Model file for the job. Use its own axes, mm. Face numbers are marked on the shaded views. A direction names the side the tool comes from. Round coordinates to 2 decimals unless told otherwise and drop trailing zeros. Loops run counter-clockwise (first coordinate to the right, second up) from the corner with the lowest first, then second, coordinate; pieces in that order, holes last. Notation, with made-up numbers: (77.25, -7) -> (89.25, -7) arc R11 cw to (89.25, 3) -> close; hole circle Ø5 at (76, 31.5). An arc over 180 degrees is marked (long way). Use a Markdown table: item, result.
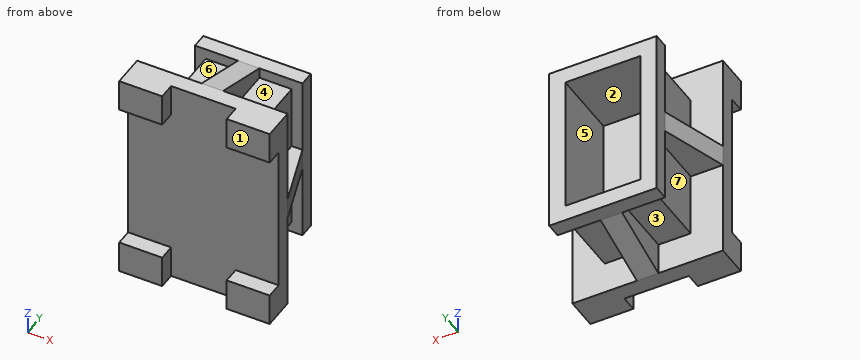
from build123d import *

# Parameters (mm, degrees)
SKETCH2_W           = 140
SKETCH2_H           = 200
BOSS_EXTRUDE1_DEPTH = 30
SKETCH3_W           = 60
SKETCH3_H           = 15
CUT_EXTRUDE1_DEPTH  = 215.00934559
SKETCH4_W           = 140
SKETCH4_H           = 15
CUT_EXTRUDE2_DEPTH  = 175.642491966
SKETCH6_W           = 80
SKETCH6_H           = 140
BOSS_EXTRUDE2_DEPTH = 61
SKETCH12_W          = 100
SKETCH12_H          = 160
SKETCH12_W_2        = 70
SKETCH12_H_2        = 130
BOSS_EXTRUDE3_DEPTH = 14
SKETCH15_W          = 70
SKETCH15_H          = 130
CUT_EXTRUDE3_DEPTH  = 50
BOSS_EXTRUDE4_DEPTH = 10
BOSS_EXTRUDE5_DEPTH = 10


with BuildPart() as part:
    # Sketch2 → Boss-Extrude1 (new body)
    with BuildSketch(Plane(origin=(0, 0, 0), x_dir=(1, 0, 0), z_dir=(0, 1, 0))):
        Rectangle(SKETCH2_W, SKETCH2_H)
    extrude(amount=BOSS_EXTRUDE1_DEPTH)

    # Sketch3 → Cut-Extrude1 (cut, through all)
    with BuildSketch(Plane.XY.offset(100)):
        with Locations((0, 7.5)):
            Rectangle(SKETCH3_W, SKETCH3_H)
    extrude(amount=-CUT_EXTRUDE1_DEPTH, mode=Mode.SUBTRACT)

    # Sketch4 → Cut-Extrude2 (cut, through all)
    with BuildSketch(Plane(origin=(70, 0, 0), x_dir=(0, 0, -1), z_dir=(1, 0, 0))):
        with Locations((0, 7.5)):
            Rectangle(SKETCH4_W, SKETCH4_H)
    extrude(amount=-CUT_EXTRUDE2_DEPTH, mode=Mode.SUBTRACT)

    # Sketch6 → Boss-Extrude2 (add)
    with BuildSketch(Plane(origin=(0, 30, 0), x_dir=(1, 0, 0), z_dir=(0, 1, 0))):
        Rectangle(SKETCH6_W, SKETCH6_H)
    extrude(amount=BOSS_EXTRUDE2_DEPTH)

    # Sketch12 → Boss-Extrude3 (add)
    with BuildSketch(Plane(origin=(0, 91, 0), x_dir=(1, 0, 0), z_dir=(0, 1, 0))):
        Rectangle(SKETCH12_W, SKETCH12_H)
        Rectangle(SKETCH12_W_2, SKETCH12_H_2, mode=Mode.SUBTRACT)
    extrude(amount=BOSS_EXTRUDE3_DEPTH)

    # Sketch15 → Cut-Extrude3 (cut)
    with BuildSketch(Plane(origin=(0, 91, 0), x_dir=(1, 0, 0), z_dir=(0, 1, 0))):
        Rectangle(SKETCH15_W, SKETCH15_H)
    extrude(amount=-CUT_EXTRUDE3_DEPTH, mode=Mode.SUBTRACT)

    # Sketch23 → Boss-Extrude4 (add, symmetric)
    with BuildSketch(Plane.XY):
        Polygon((-50, 91), (-70, 30), (-40, 30), (-40, 91), align=None)
    boss_extrude4 = extrude(amount=BOSS_EXTRUDE4_DEPTH, both=True)

    # Mirror1: Boss-Extrude4 across plane
    add(boss_extrude4.mirror(Plane(origin=(0, 0, 0), x_dir=(0, 0, 1), z_dir=(1, 0, 0))))

    # Sketch24 → Boss-Extrude5 (add, symmetric)
    with BuildSketch(Plane(origin=(0, 0, 0), x_dir=(0, 0, -1), z_dir=(1, 0, 0))):
        Polygon((-80, 91), (-100, 30), (-70, 30), (-70, 91), align=None)
    boss_extrude5 = extrude(amount=BOSS_EXTRUDE5_DEPTH, both=True)

    # Mirror2: Boss-Extrude5 across plane
    add(boss_extrude5.mirror(Plane.XY))


solid = part.part
Q1. Drill centre lines: L1, parallel to Y at x = 33, z = -73; L2, parallel to Z at x = 17, y = 47; L3, parallel to X at y = 62, z = 25. Where is each one in solid material? Low to high. Write a range as from..to.
Results list:
| item | result |
|---|---|
| L1 | y = 0..30, 91..105 |
| L2 | z = -70..-65, 65..70 |
| L3 | x = -40..-35, 35..40 |
Q2. Pull direction Z, two halves, no side cores. Call the marked faces 1, 2 and 3: released by +Z, released by -Z, zero draft, split by the parting line, or undercut.
Results list:
| item | result |
|---|---|
| face 1 | zero draft |
| face 2 | undercut |
| face 3 | released by -Z |
Q3. Band-saw the part on B-B, the plane z = -67.5. Give the cut face in (x, y).
Results list:
| item | result |
|---|---|
| outline | (-70, 15) -> (70, 15) -> (70, 30) -> (40, 30) -> (40, 91) -> (50, 91) -> (50, 105) -> (-50, 105) -> (-50, 91) -> (-40, 91) -> (-40, 30) -> (-70, 30) -> close |
Q4. Band-saw the part on A-A, the plane y = 96.5. Give the cut face in (x, z).
Results list:
| item | result |
|---|---|
| outline | (-50, -80) -> (50, -80) -> (50, 80) -> (-50, 80) -> close; hole (-35, -65) -> (35, -65) -> (35, 65) -> (-35, 65) -> close |
Q5. Band-saw the part on D-D, the plane x = 15. Give the cut face in (y, z), plus the area to 3 significant figures.
Results list:
| item | result |
|---|---|
| outline | (15, -100) -> (30, -100) -> (30, -70) -> (91, -70) -> (91, -80) -> (105, -80) -> (105, -65) -> (41, -65) -> (41, 65) -> (105, 65) -> (105, 80) -> (91, 80) -> (91, 70) -> (30, 70) -> (30, 100) -> (15, 100) -> close |
| area | 5,460 mm² |
Q6. Tool access for the marked faces 4, 5, 6 and 7: list every direction of +Z, -Z, +X, -X, +Y, -Y with a clear straight run to the whole face (end or side of a thin tool).
Results list:
| item | result |
|---|---|
| face 4 | +Z, +X |
| face 5 | +Y |
| face 6 | +Z, -X |
| face 7 | -Z, -X |
Q7. Band-saw the part on C-C, the plane x = -2. Give the cut face in (y, z).
Results list:
| item | result |
|---|---|
| outline | (15, -100) -> (30, -100) -> (91, -80) -> (105, -80) -> (105, -65) -> (41, -65) -> (41, 65) -> (105, 65) -> (105, 80) -> (91, 80) -> (30, 100) -> (15, 100) -> close |
Q8. Flat gauge pins, fed straight in: pin 1 (8 mm diameter, centred on y = 63.5, z = 42.5, fed in from +X); pin 2 (4 mm diameter, centred on x = 29, z = -7.5, fed in from +Y); pin 3 (2 mm diameter, centred on x = 46, z = -54.5, fed in from -Y). Where does each tip first touch, or does it go through?
Results list:
| item | result |
|---|---|
| pin 1 | stops at x = 40 |
| pin 2 | stops at y = 41 |
| pin 3 | stops at y = 15 |
